Work out the finished part from the listing and answer in its coordinate system (mm). A direction names the side the tool comes from. Round coordinates to 2 decimals unless told otherwise and drop trailing zeros. Loops run counter-clockwise (first coordinate to the right, second up) from the corner with the lowest first, then second, coordinate; pieces in that order, holes last. Notation, with made-up numbers: M 86.5,57.25 L 141.5,57.25 A20 ccw 141.5,96.25 Z; hole C 34,72 d1. An arc over 180 degrees is marked long. One line per item, written item: value.
```python
from build123d import *

# Parameters (mm, degrees)
SKETCH2_R               = 18
BOSS_EXTRUDE1_DEPTH     = 30
SKETCH4_W               = 36
SKETCH4_H               = 55
BOSS_EXTRUDE2_DEPTH     = 3
CUT_EXTRUDE1_DEPTH      = 3
CUT_EXTRUDE1_DEPTH_BACK = 60
SKETCH3_R               = 3
SKETCH6_W               = 36
SKETCH6_H               = 47
BOSS_EXTRUDE3_DEPTH     = 3
BOSS_EXTRUDE4_DEPTH     = 5
SKETCH8_W               = 36
SKETCH8_H               = 3
BOSS_EXTRUDE5_DEPTH     = 7.5


with BuildPart() as part:
    # Sketch2 → Boss-Extrude1 (new body)
    with BuildSketch(Plane.XY):
        Circle(SKETCH2_R)
    extrude(amount=BOSS_EXTRUDE1_DEPTH)

    # Sketch4 → Boss-Extrude2 (add)
    with BuildSketch(Plane.XY.offset(30)):
        with Locations((0, 9.5)):
            Rectangle(SKETCH4_W, SKETCH4_H)
    extrude(amount=BOSS_EXTRUDE2_DEPTH)

    # Sketch3 → Cut-Extrude1 (cut, two sides: drawn at the far end of the back side and taken through both)
    with BuildSketch(Plane.XY.offset(30).offset(-CUT_EXTRUDE1_DEPTH_BACK)):
        Circle(SKETCH3_R)
    extrude(amount=CUT_EXTRUDE1_DEPTH + CUT_EXTRUDE1_DEPTH_BACK, mode=Mode.SUBTRACT)

    # Sketch6 → Boss-Extrude3 (add)
    with BuildSketch(Plane(origin=(0, 37, 0), x_dir=(1, 0, 0), z_dir=(0, 1, 0))):
        with Locations((0, -56.5)):
            Rectangle(SKETCH6_W, SKETCH6_H)
    extrude(amount=-BOSS_EXTRUDE3_DEPTH)

    # Sketch7 → Boss-Extrude4 (add)
    with BuildSketch(Plane.XY.offset(80)):
        Polygon((18, 34), (18, 12.5), (-18, 12.5), (-18, 34), (-18, 37), (18, 37), align=None)
    extrude(amount=BOSS_EXTRUDE4_DEPTH)

    # Sketch8 → Boss-Extrude5 (add)
    with BuildSketch(Plane.XY.offset(85)):
        with Locations((0, 14)):
            Rectangle(SKETCH8_W, SKETCH8_H)
    extrude(amount=BOSS_EXTRUDE5_DEPTH)


solid = part.part
```
1) Find section D-D (x = 8). Give the vertices of the cut face in (y, z).
Check values:
outline: M -18,30 L -16.12,30 L -16.12,0 L 16.12,0 L 16.12,30 L 37,30 L 37,85 L 15.5,85 L 15.5,92.5 L 12.5,92.5 L 12.5,80 L 34,80 L 34,33 L -18,33 Z
2) Find section B-B (x = 2). Give the vertices of the cut face in (y, z).
Check values:
outline: M -18,30 L -17.89,30 L -17.89,0 L -2.24,0 L -2.24,33 L -18,33 Z; M 2.24,0 L 17.89,0 L 17.89,30 L 37,30 L 37,85 L 15.5,85 L 15.5,92.5 L 12.5,92.5 L 12.5,80 L 34,80 L 34,33 L 2.24,33 Z
3) The mould has two halves that part along X. Classify faces 6 (the face through (0, -18, 31)), 7 (the face through (-3, 0, 16)), 8 (the face through (-2.343, 17.847, 14.79)): +X half, -X half, draft (parallel to the pull), parting line (faces both ways), or undercut.
Check values:
face 6: draft
face 7: undercut
face 8: parting line
4) Find the intervals of material crossed by probe 1 along Y at (x, z) = (0, 12); probe 2 along Z at (x, y) = (9, 29.5); probe 3 along Y at (x, z) = (6, 63.5), in increasing order. Write a range as from..to.
Check values:
probe 1: -18..-3, 3..18
probe 2: 30..33, 80..85
probe 3: 34..37
5) Each of these flat-tipped pins is pushed along its axis until it touches: pin 1 (12 mm diameter, centred on x = -11.5, z = 68, fed in from -Y); pin 2 (6 mm diameter, centred on x = 5, z = 89, fed in from +Y); pin 3 (18 mm diameter, centred on x = -1, y = 1.5, fed in from +Z). Where does it stop, or does it pass through?
Check values:
pin 1: y = 34
pin 2: y = 15.5
pin 3: z = 33
6) For faces 1 (the face through (14, -14, 30)), 2 (the face through (0, 26, 85)), 3 (the face through (0, 34, 56)), 4 (the face through (0, 12.5, 86)), 5 (the face through (-14, -14, 30)), determine the directions among +Z, -Z, +X, -X, +Y, -Y from which every point of the face is accessible in a straight line to the end or side of a thin tool.
Check values:
face 1: -Z, +X, -Y
face 2: +Z, +X, -X, +Y
face 3: +X, -X, -Y
face 4: +Z, +X, -X, -Y
face 5: -Z, -X, -Y
7) Find section C-C (z = 20). Give the vertices of the cut face in (x, y).
Check values:
outline: C 0,0 d36; hole C 0,0 d6
8) Find section A-A (y = 32). Give the vertices of the cut face in (x, z).
Check values:
outline: M -18,30 L 18,30 L 18,33 L -18,33 Z; M -18,80 L 18,80 L 18,85 L -18,85 Z
